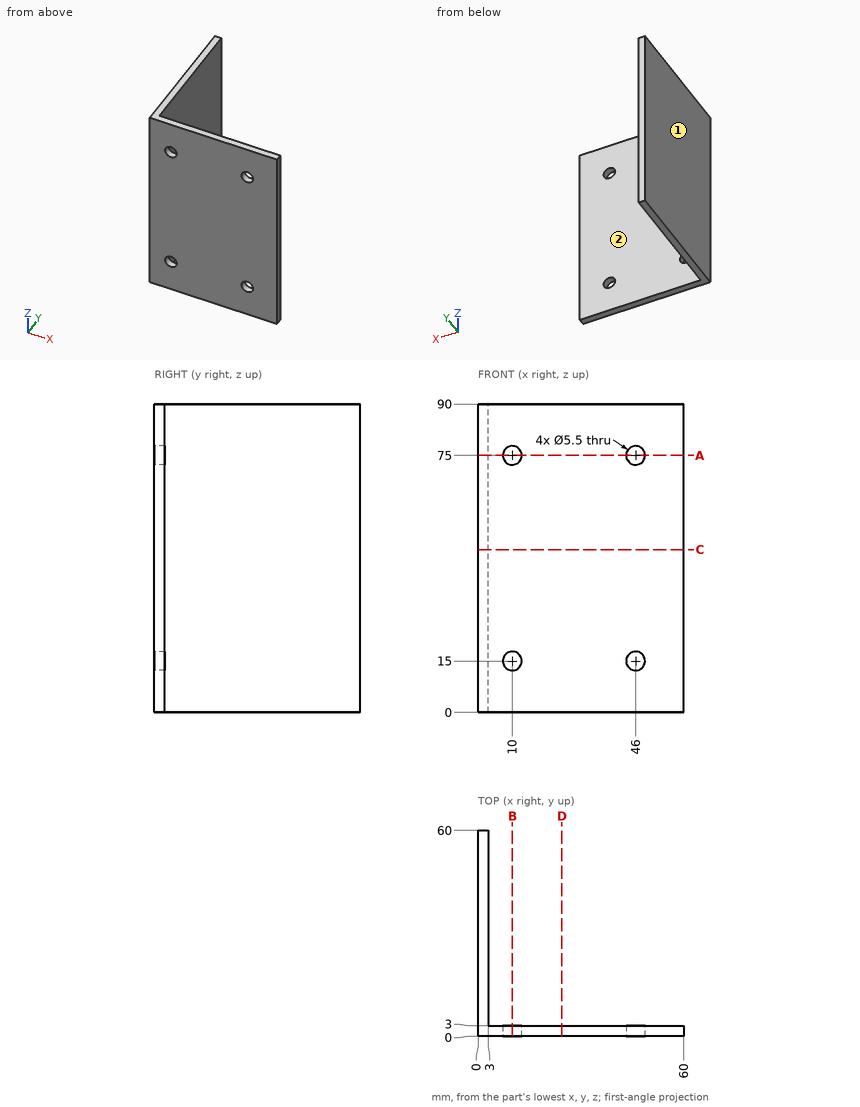
Answer from the drawing. Dimensions are ordinates in mm from the lowest x, y and z of the part. A direction names the side the tool comes from. Coordinates: 2 decimals unless noted, no trailing zeros. Loops run counter-clockwise (first coordinate to the right, second up) from the corner with the lowest first, then second, coordinate; pieces in that order, holes last. Notation, with made-up numbers: (25, 44) -> (52, 44) arc R17 cw to (52, 64) -> close; hole circle Ø4 at (35, 9). An arc over 180 degrees is marked (long way). Answer in a Markdown table with one row per item.
Item 1: Each of these flat-tipped pins is pushed along its axis until it touches: P1, Ø5, axis at y = 48.5, z = 49.5, coming from the +X side; P2, Ø1, axis at y = 25, z = 38.5, coming from the -X side; P3, Ø5, axis at x = 46, z = 15, coming from the -Y side; P4, Ø1.5, axis at x = 19, z = 23, coming from the +Y side. Where does it stop, or does it pass through?
Returned:
| item | result |
|---|---|
| P1 | stops at x = 3 |
| P2 | stops at x = 0 |
| P3 | passes through |
| P4 | stops at y = 3 |
Item 2: A cutting plane is placed at A-A on z = 75. Determine the outline of the cut face in (x, y).
Returned:
| item | result |
|---|---|
| outline | (0, 0) -> (7.25, 0) -> (7.25, 3) -> (3, 3) -> (3, 60) -> (0, 60) -> close; (12.75, 0) -> (43.25, 0) -> (43.25, 3) -> (12.75, 3) -> close; (48.75, 0) -> (60, 0) -> (60, 3) -> (48.75, 3) -> close |
Item 3: A cutting plane is placed at B-B on x = 10. Determine the outline of the cut face in (y, z).
Returned:
| item | result |
|---|---|
| outline | (0, 0) -> (3, 0) -> (3, 12.25) -> (0, 12.25) -> close; (0, 17.75) -> (3, 17.75) -> (3, 72.25) -> (0, 72.25) -> close; (0, 77.75) -> (3, 77.75) -> (3, 90) -> (0, 90) -> close |
Item 4: A cutting plane is placed at C-C on z = 47.5. Determine the outline of the cut face in (x, y), plus the area to 3 significant figures.
Returned:
| item | result |
|---|---|
| outline | (0, 0) -> (60, 0) -> (60, 3) -> (3, 3) -> (3, 60) -> (0, 60) -> close |
| area | 351 mm^2 |
Item 5: For the marked faces 1 and 2, determine the directions among +Z, -Z, +X, -X, +Y, -Y from which every point of the face is accessible in a straight line to the end or side of a thin tool.
Returned:
| item | result |
|---|---|
| face 1 | +Z, -Z, -X, +Y, -Y |
| face 2 | +Z, -Z, +X, +Y |
Item 6: A cutting plane is placed at D-D on x = 24.5. Determine the outline of the cut face in (y, z), plus the area to 3 significant figures.
Returned:
| item | result |
|---|---|
| outline | (0, 0) -> (3, 0) -> (3, 90) -> (0, 90) -> close |
| area | 270 mm^2 |
Item 7: Straight lines are drawn through the part: line 1 along Z through (x, y) = (10, 1.35); line 2 along Y through (x, z) = (15.5, 68). For each, find the intervals that lie inside material, in ascending order. Write a range as [from, to].
Returned:
| item | result |
|---|---|
| line 1 | z = [0, 12.25], [17.75, 72.25], [77.75, 90] |
| line 2 | y = [0, 3] |
